```python
from build123d import *

# Parameters (mm, degrees)
F1_DEPTH = 7.62
F2_R     = 5.08
F4_DEPTH = 45.72
F6_DEPTH = 25.4
F7_W     = 43.18
F7_H     = 3.175
F8_DEPTH = 36.576
F9_R     = 8.0330542074


with BuildPart() as f1:
    # F0 (on Top) → F1 (new body)
    with BuildSketch(Plane.XY):
        with BuildLine():
            ThreePointArc((-19.05, 16.5915609938), (-20.5766435406, 20.2772045344), (-16.891, 18.7505609938))
            Line((-16.891, 18.7505609938), (16.891, 18.7505609938))
            ThreePointArc((16.891, 18.7505609938), (19.05, 20.9095609938), (21.209, 18.7505609938))
            ThreePointArc((21.209, 18.7505609938), (20.5766435406, 17.2239174532), (19.05, 16.5915609938))
            Line((19.05, 16.5915609938), (19.05, 0))
            Line((19.05, 0), (52.1362312138, 0))
            Line((52.1362312138, 0), (52.1362312138, 51.7165437341))
            Line((52.1362312138, 51.7165437341), (-52.0691390008, 51.7165437341))
            Line((-52.0691390008, 51.7165437341), (-52.0691390008, 0))
            Line((-52.0691390008, 0), (-19.05, 0))
            Line((-19.05, 0), (-19.05, 16.5915609938))
        make_face()
        with BuildLine():
            Line((-19.05, -16.5915609938), (-19.05, 0))
            Line((-19.05, 0), (-52.0691390008, 0))
            ThreePointArc((-52.0691390008, 0), (0.0335461065, -52.1026851073), (52.1362312138, 0))
            Line((52.1362312138, 0), (19.05, 0))
            Line((19.05, 0), (19.05, -16.5915609938))
            ThreePointArc((19.05, -16.5915609938), (20.5766435406, -17.2239174532), (21.209, -18.7505609938))
            ThreePointArc((21.209, -18.7505609938), (19.3524205753, -20.8882753797), (16.975722746, -19.3494390062))
            Line((16.975722746, -19.3494390062), (-16.975722746, -19.3494390062))
            ThreePointArc((-16.975722746, -19.3494390062), (-20.775435978, -20.0483096928), (-19.05, -16.5915609938))
        make_face()
        with BuildLine():
            Line((16.891, 18.7505609938), (-16.891, 18.7505609938))
            ThreePointArc((-16.891, 18.7505609938), (-17.5233564594, 17.2239174532), (-19.05, 16.5915609938))
            Line((-19.05, 16.5915609938), (-19.05, 0))
            Line((-19.05, 0), (19.05, 0))
            Line((19.05, 0), (19.05, 16.5915609938))
            ThreePointArc((19.05, 16.5915609938), (17.5233564594, 17.2239174532), (16.891, 18.7505609938))
        make_face()
        with BuildLine():
            Line((19.05, 0), (-19.05, 0))
            Line((-19.05, 0), (-19.05, -16.5915609938))
            ThreePointArc((-19.05, -16.5915609938), (-17.5233564594, -17.2239174532), (-16.891, -18.7505609938))
            ThreePointArc((-16.891, -18.7505609938), (-16.9122856141, -19.0529815691), (-16.975722746, -19.3494390062))
            Line((-16.975722746, -19.3494390062), (16.975722746, -19.3494390062))
            ThreePointArc((16.975722746, -19.3494390062), (17.324564022, -17.4528122949), (19.05, -16.5915609938))
            Line((19.05, -16.5915609938), (19.05, 0))
        make_face()
    extrude(amount=F1_DEPTH)

    # F2
    f2_edges = [f1.edges().sort_by_distance(p)[0] for p in [
        (0.033546, -52.102685, 7.62),
    ]]
    fillet(f2_edges, radius=F2_R)

    # F3 (on face) → F4 (join)
    with BuildSketch(Plane.XY.offset(7.62)):
        Polygon((46.1304020137, 23.6876853067), (2.9504020137, 23.6876853067), (2.9504020137, 57.9776853067), (2.9504020137, 60.2722298354), (0.6876643932, 60.2722298354), (0.6876643932, 21.3931407779), (48.3931396341, 21.3931407779), (48.3931396341, 60.2722298354), (46.1304020137, 60.2722298354), (46.1304020137, 57.9776853067), align=None)
    extrude(amount=F4_DEPTH)

    # F5 (on face) → F6 (cut)
    with BuildSketch(Plane.XZ.offset(-21.3931407779)):
        with BuildLine():
            ThreePointArc((6.5425638128, 44.8215786717), (8.7015638128, 42.6625786717), (10.8605638128, 44.8215786717))
            ThreePointArc((10.8605638128, 44.8215786717), (10.2282073534, 46.3482222123), (8.7015638128, 46.9805786717))
            ThreePointArc((8.7015638128, 46.9805786717), (7.1749202722, 46.3482222123), (6.5425638128, 44.8215786717))
        make_face()
        with BuildLine():
            ThreePointArc((24.9343014333, 39.9498267307), (17.1214786079, 21.0880039054), (35.9833014333, 28.9008267307))
            ThreePointArc((35.9833014333, 28.9008267307), (32.7471242586, 36.7136495561), (24.9343014333, 39.9498267307))
        make_face()
        with BuildLine():
            ThreePointArc((41.1670390537, 46.9805786717), (39.6403955132, 43.2949351311), (43.3260390537, 44.8215786717))
            ThreePointArc((43.3260390537, 44.8215786717), (42.6936825943, 46.3482222123), (41.1670390537, 46.9805786717))
        make_face()
        with BuildLine():
            ThreePointArc((41.1670390537, 10.8210747898), (42.6936825943, 11.4534312492), (43.3260390537, 12.9800747898))
            ThreePointArc((43.3260390537, 12.9800747898), (39.6403955132, 14.5067183303), (41.1670390537, 10.8210747898))
        make_face()
        with BuildLine():
            ThreePointArc((6.5425638128, 12.9800747898), (7.1749202722, 11.4534312492), (8.7015638128, 10.8210747898))
            ThreePointArc((8.7015638128, 10.8210747898), (10.2282073534, 11.4534312492), (10.8605638128, 12.9800747898))
            ThreePointArc((10.8605638128, 12.9800747898), (8.7015638128, 15.1390747898), (6.5425638128, 12.9800747898))
        make_face()
    extrude(amount=-F6_DEPTH, mode=Mode.SUBTRACT)

    # F7 (on face) → F8 (join)
    with BuildSketch(Plane(origin=(0, 23.6876853067, 0), x_dir=(-1, 0, 0), z_dir=(0, 1, 0))):
        with Locations((-24.5404020137, 51.7525)):
            Rectangle(F7_W, F7_H)
    extrude(amount=F8_DEPTH)

    # F9
    f9_edges = [f1.edges().sort_by_distance(p)[0] for p in [
        (47.261771, 60.27223, 7.62),
        (1.819033, 60.27223, 7.62),
    ]]
    fillet(f9_edges, radius=F9_R)


solid = f1.part
```
Build history of the part. All positions in model axes, mm. A direction names the side the tool comes from. Round coordinates to 2 decimals unless told otherwise and drop trailing zeros. Loops run counter-clockwise (first coordinate to the right, second up) from the corner with the lowest first, then second, coordinate; pieces in that order, holes last.
Item 1: Pin check, flat tips, straight feed: P1, Ø10, axis at x = 19.5, z = 47, coming from the -Y side; P2, Ø2.5, axis at x = -5, z = 5.5, coming from the +Y side; P3, Ø10, axis at x = 16, z = 31.5, coming from the +Y side. Stop position of each tip, or through.
Item 2: Saw through at D-D (z = 36). List the corners of the cut face in (x, y), then the cut area to 3 significant figures.
Item 3: Drill centre lines: line 1 along X through (y, z) = (44, 23); line 2 along Z through (x, y) = (43, 39) (3 decimals); line 3 along Y through (x, z) = (-19.05, 3). Where is each one in solid material? Low to high.
Item 4: Saw through at A-A (z = 22). List the corners of the cut face in (x, y), then the cut area to 3 significant figures.
Item 5: Saw through at B-B (y = 45.5). List the corners of the cut face in (x, z) (3 decimals).
Item 6: Which spindle directions (+Z, -Z, +X, -X, +Y, -Y) get a long thin tool onto all of the face, cutting with end or side? Do faces 4 (the face through (0.688, 41, 30)), 5 (the face through (24.2, 21.393, 40.3)), 6 (the face through (2.95, 42, 30)). Say none if no direction does.
Item 7: Two-plate mould, pull along X, no slides. Class faces 1 (the face through (-52.069, 26, 1)), 2 (the face through (-1, 1, 0)), 3 (the face through (25, 42, 50.165)): released by +X, released by -X, zero draft, split by the parting line, or undercut.
Worked answers:
1. P1: stops at y = 21.39
1. P2: stops at y = 51.72
1. P3: stops at y = 23.69
2. outline: (0.69, 21.39) - (16.47, 21.39) - (16.47, 23.69) - (2.95, 23.69) - (2.95, 60.27) - (0.69, 60.27) - close; (33.4, 21.39) - (48.39, 21.39) - (48.39, 60.27) - (46.13, 60.27) - (46.13, 23.69) - (33.4, 23.69) - close
2. area: 236 mm2
3. line 1: x = 0.69 to 2.95, 46.13 to 48.39
3. line 2: z = 0 to 7.62, 50.165 to 53.34
3. line 3: y = -48.46 to -20.91, -16.59 to 16.59, 20.91 to 51.72
4. outline: (0.69, 21.39) - (16.31, 21.39) - (16.31, 23.69) - (2.95, 23.69) - (2.95, 60.27) - (0.69, 60.27) - close; (33.56, 21.39) - (48.39, 21.39) - (48.39, 60.27) - (46.13, 60.27) - (46.13, 23.69) - (33.56, 23.69) - close
4. area: 235 mm2
5. outline: (-52.069, 0) - (52.136, 0) - (52.136, 2.54) arc R5.08 ccw to (47.056, 7.62) - (48.393, 7.62) - (48.393, 53.34) - (0.688, 53.34) - (0.688, 7.62) - (-46.989, 7.62) arc R5.08 ccw to (-52.069, 2.54) - close; hole (2.95, 7.62) - (46.13, 7.62) - (46.13, 50.165) - (2.95, 50.165) - close
6. face 4: +Z, -X, +Y, -Y
6. face 5: +Z, +X, -X, -Y
6. face 6: +Y
7. face 1: released by -X
7. face 2: zero draft
7. face 3: undercut
